The drawing under review shows one solid part. Ordinate dimensions are in mm from its lowest x, y, z. A direction names the side the tool comes from. Round coordinates to 2 decimals unless told otherwise and drop trailing zeros. Order: outer loops, then holes, each group sorted by start corner. A loop starts at its lowest first (then second) coordinate and runs counter-clockwise, first axis right, second up.
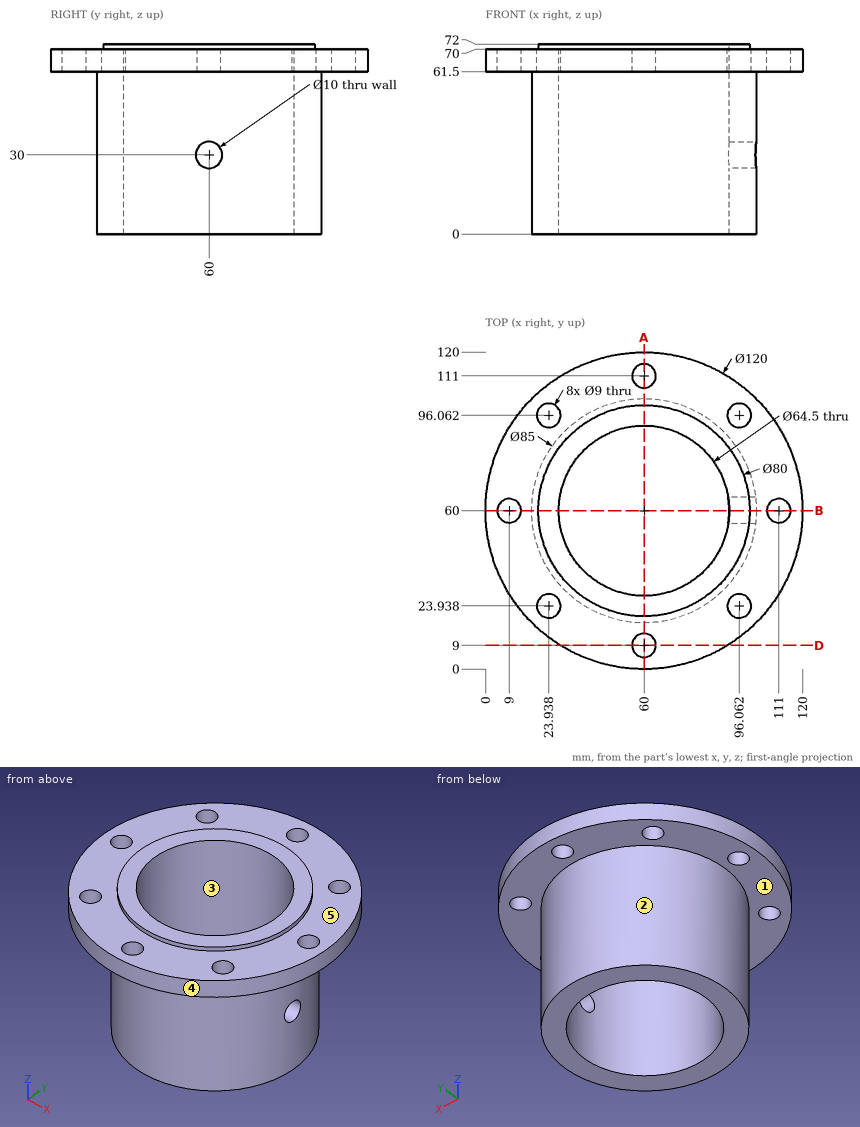
Q1. Take a section at A-A, the plane x = 60. State the section outline as (y, z) points.
Q2. Mouldability with a two-part tool opening along Y and no side actions: class the marked faces 1, 2 and 3 as +Y half, -Y half, draft (parallel to the pull), parting line (faces both ways), or undercut.
Q3. Take a section at D-D, the plane y = 9. State the section outline as (x, z) points.
Q4. Take a section at B-B, the plane y = 60. State the section outline as (x, z) points, plus the area to 3 significant figures.
Q5. Tool access review of the marked faces 4 and 5: name each direction out of +Z, -Z, +X, -X, +Y, -Y from which nothing blocks a thin tool from reaching the whole face with its end or side.
Q6. Clearance check with flat-ended pins moving along their axes: pin 1 (4 mm diameter, centred on y = 41.5, z = 59, fed in from -X); pin 2 (8 mm diameter, centred on y = 58, z = 42.5, fed in from -X); pin 3 (8 mm diameter, centred on y = 91, z = 8, fed in from -X). State where each tip first meets the part, or that it passes through.
Q7. Wall thickness on line 1 (Z direction, x = 91, y = 100.5); line 2 (X direction, y = 111, z = 67) (1 decimal); line 3 (Y direction, x = 37.5, z = 24.5) (1 decimal): over which ranges is each line inside the solid? List them lowest first.
Working result:
1. outline: (0, 61.5) - (4.5, 61.5) - (4.5, 70) - (0, 70) - close; (13.5, 61.5) - (17.5, 61.5) - (17.5, 0) - (27.75, 0) - (27.75, 72) - (20, 72) - (20, 70) - (13.5, 70) - close; (92.25, 0) - (102.5, 0) - (102.5, 61.5) - (106.5, 61.5) - (106.5, 70) - (100, 70) - (100, 72) - (92.25, 72) - close; (115.5, 61.5) - (120, 61.5) - (120, 70) - (115.5, 70) - close
2. face 1: draft
2. face 2: parting line
2. face 3: undercut
3. outline: (28.39, 61.5) - (55.5, 61.5) - (55.5, 70) - (28.39, 70) - close; (64.5, 61.5) - (91.61, 61.5) - (91.61, 70) - (64.5, 70) - close
4. outline: (0, 61.5) - (4.5, 61.5) - (4.5, 70) - (0, 70) - close; (13.5, 61.5) - (17.5, 61.5) - (17.5, 0) - (27.75, 0) - (27.75, 72) - (20, 72) - (20, 70) - (13.5, 70) - close; (92.25, 0) - (102.5, 0) - (102.5, 25) - (92.25, 25) - close; (92.25, 35) - (102.5, 35) - (102.5, 61.5) - (106.5, 61.5) - (106.5, 70) - (100, 70) - (100, 72) - (92.25, 72) - close; (115.5, 61.5) - (120, 61.5) - (120, 70) - (115.5, 70) - close
4. area: 1,510 mm2
5. face 4: +Z, -Z
5. face 5: +Z
6. pin 1: stops at x = 20.83
6. pin 2: stops at x = 17.5
6. pin 3: stops at x = 27.18
7. line 1: z = 61.5 to 70
7. line 2: x = 28.4 to 55.5, 64.5 to 91.6
7. line 3: y = 23.9 to 36.9, 83.1 to 96.1
